```python
from build123d import *

# Parameters (mm, degrees)
FILLET1_R = 0.381
FILLET2_R = 0.127


with BuildPart() as part:
    # Sketch1 → Revolve1 (revolve)
    with BuildSketch(Plane.XY):
        Polygon((1.651, 0), (5.207, 0), (5.207, 1.667634761), (4.572, 1.667634761), (4.5212, 1.032634761), (4.7625, 1.032634761), (4.7625, 0.49747982), (1.651, 0.49747982), align=None)
    revolve(axis=Axis((0, -34.221434911, 0), (0, 1, 0)))

    # Fillet1
    fillet1_edges = [part.edges().sort_by_distance(p)[0] for p in [
        (-5.207, 0, 0),
    ]]
    fillet(fillet1_edges, radius=FILLET1_R)

    # Fillet2
    fillet2_edges = [part.edges().sort_by_distance(p)[0] for p in [
        (-1.651, 0.49747982, 0),
        (-4.7625, 0.49747982, 0),
        (-4.572, 1.667634761, 0),
        (-5.207, 1.667634761, 0),
    ]]
    fillet(fillet2_edges, radius=FILLET2_R)


solid = part.part
```
Source: CAD feature listing. Evaluate the final solid. Frame: model axes, mm. A direction names the side the tool comes from. Coordinates: 2 decimals unless noted, no trailing zeros. Loops run counter-clockwise (first coordinate to the right, second up) from the corner with the lowest first, then second, coordinate; pieces in that order, holes last. Notation, with made-up numbers: M 33,66 L 70,66 A3 ccw 70,70 Z; hole C -8,41 d10. An arc over 180 degrees is marked long. Use CSV: the item, a comma, the result in double quotes.
(1) Draft query along X for faces 1 (the face through (0, 0.497, 2)), 2 (the face through (4.967, 0.969, -1.564)), 3 (the face through (-2, 0, 0)). Return one class per face: pulls with the +X half, pulls with the -X half, needs draft (parallel to the pull), parting line crosses it, or undercut.
Answers follow:
face 1,"undercut"
face 2,"parting line crosses it"
face 3,"needs draft"
(2) Reachability of faces 4 (the face through (1.525, 0.183, 0.632)), 5 (the face through (-3.78, 0.83, 2.9)) from +Z, -Z, +X, -X, +Y, -Y: full face, straight path, thin tool, end or side. Return the list, or none.
Answers follow:
face 4,"+Y, -Y"
face 5,"none"
(3) Cut plane C-C on y = 0.2. Return loops of the section in (x, z).
Answers follow:
outline,"C 0,0 d10.32; hole C 0,0 d3.3"
(4) Line query: line 1 (X direction, y = 0.85, z = 0); line 2 (Z direction, x = 0, y = 0.1). Output: solid intervals per line, ascending. Write a range as [from, to].
Answers follow:
line 1,"[-5.21, -4.76], [4.76, 5.21]"
line 2,"[-5.08, -1.65], [1.65, 5.08]"
(5) Cut plane A-A on z = 0. Return loops of the section in (x, y).
Answers follow:
outline,"M -5.21,0.38 A0.38 ccw -4.83,0 L -1.65,0 L -1.65,0.37 A0.13 ccw -1.78,0.5 L -4.64,0.5 A0.13 cw -4.76,0.62 L -4.76,1.03 L -4.52,1.03 L -4.56,1.55 A0.13 ccw -4.69,1.67 L -5.08,1.67 A0.13 ccw -5.21,1.54 Z; M 1.65,0 L 4.83,0 A0.38 ccw 5.21,0.38 L 5.21,1.54 A0.13 ccw 5.08,1.67 L 4.69,1.67 A0.13 ccw 4.56,1.55 L 4.52,1.03 L 4.76,1.03 L 4.76,0.62 A0.13 cw 4.64,0.5 L 1.78,0.5 A0.13 ccw 1.65,0.37 Z"
(6) Cut plane B-B on x = 0. Return loops of the section in (y, z), and give its area (3 significant figures).
Answers follow:
outline,"M 0,-4.83 A0.38 ccw 0.38,-5.21 L 1.54,-5.21 A0.13 ccw 1.67,-5.08 L 1.67,-4.69 A0.13 ccw 1.55,-4.56 L 1.03,-4.52 L 1.03,-4.76 L 0.62,-4.76 A0.13 cw 0.5,-4.64 L 0.5,-1.78 A0.13 ccw 0.37,-1.65 L 0,-1.65 Z; M 0,1.65 L 0.37,1.65 A0.13 ccw 0.5,1.78 L 0.5,4.64 A0.13 cw 0.62,4.76 L 1.03,4.76 L 1.03,4.52 L 1.55,4.56 A0.13 ccw 1.67,4.69 L 1.67,5.08 A0.13 ccw 1.54,5.21 L 0.38,5.21 A0.38 ccw 0,4.83 Z"
area,"4.78 mm²"
(7) Contact query for a flat-ended pin moving along its axis: pin 1 (1.5 mm diameter, centred on x = -0.5, z = 1.5, fed in from +Y). Output: stop coordinate, or through.
Answers follow:
pin 1,"y = 0.5"
(8) Cut plane D-D on y = 1.3. Return loops of the section in (x, z).
Answers follow:
outline,"C 0,0 d10.41; hole C 0,0 d9.09"
